```python
from build123d import *

# Parameters (mm, degrees)
F0_W     = 203.2
F0_H     = 15.875
F1_DEPTH = 342.9
F3_DEPTH = 342.9
F4_W     = 15.875
F4_H     = 5.55625
F5_DEPTH = 203.2


with BuildPart() as f1:
    # F0 (on Front) → F1 (new body)
    with BuildSketch(Plane.XZ):
        with Locations((101.6, 7.9375)):
            Rectangle(F0_W, F0_H)
    extrude(amount=F1_DEPTH)

    # F2 (on face) → F3 (cut, through all)
    with BuildSketch(Plane.XZ.offset(342.9)):
        Polygon((32.54375, 5.55625), (32.54375, 0), (56.35625, 0), (56.35625, 5.55625), (53.975, 5.55625), (53.975, 3.96875), (34.925, 3.96875), (34.925, 5.55625), align=None)
        Polygon((170.65625, 5.55625), (168.275, 5.55625), (168.275, 3.96875), (149.225, 3.96875), (149.225, 5.55625), (146.84375, 5.55625), (146.84375, 0), (170.65625, 0), align=None)
    extrude(amount=-F3_DEPTH, mode=Mode.SUBTRACT)

    # F4 (on face) → F5 (cut, through all)
    with BuildSketch(Plane(origin=(0, 0, 0), x_dir=(0, -1, 0), z_dir=(-1, 0, 0))):
        with Locations((20.6375, 13.096875)):
            Rectangle(F4_W, F4_H)
        with Locations((322.2625, 13.096875)):
            Rectangle(F4_W, F4_H)
    extrude(amount=-F5_DEPTH, mode=Mode.SUBTRACT)


solid = f1.part
```
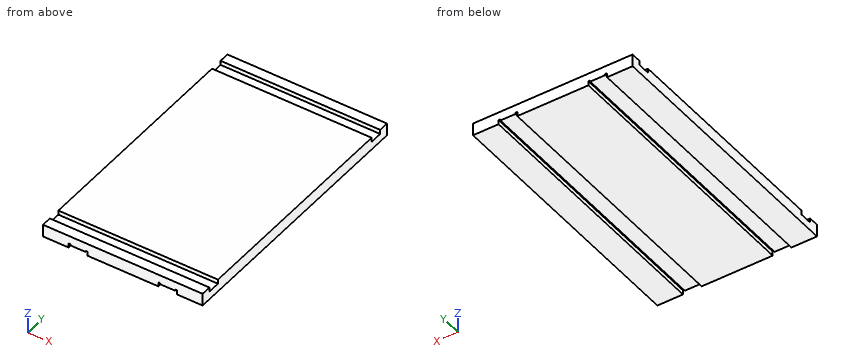
For this review, take the finished solid that the model builds, in its own axes (mm). Coordinates: 2 decimals unless noted, no trailing zeros. Write each loop counter-clockwise with the first axis right and the second up, starting at its lowest first coordinate (ties: lowest second). Pieces come first, ordered by that corner, then holes. Notation, with made-up numbers: (65, 1.5) -> (86, 1.5) arc R23 ccw to (86, 22.5) -> close; hole circle Ø9 at (47.5, -27). An arc over 180 degrees is marked (long way). Put each result on its own line as item: value.
Q1. Clearance check with flat-ended pins moving along their axes: pin 1 Ø8 at (x, y) = (114, -321) entering from +Z; pin 2 Ø1.9 at (x, y) = (54.5, -171) entering from -Z; pin 3 Ø1.9 at (x, y) = (169.5, -219) entering from -Z. State where each tip first meets the part, or that it passes through.
From the geometry:
pin 1: stops at z = 10.32
pin 2: stops at z = 3.97
pin 3: stops at z = 5.56
Q2. Wall thickness on L1, parallel to X at y = -265, z = 3; L2, parallel to X at y = -210, z = 4.25 (3 decimals); L3, parallel to Y at x = 50, z = 12.5 (3 decimals): over which ranges is each line inside the solid? List them lowest first.
From the geometry:
L1: x = 0 to 32.54, 56.36 to 146.84, 170.66 to 203.2
L2: x = 0 to 32.544, 34.925 to 53.975, 56.356 to 146.844, 149.225 to 168.275, 170.656 to 203.2
L3: y = -342.9 to -330.2, -314.325 to -28.575, -12.7 to 0
Q3. Take a section at B-B, the plane x = 154. State the section outline as (y, z) points (3 decimals).
From the geometry:
outline: (-342.9, 3.969) -> (0, 3.969) -> (0, 15.875) -> (-12.7, 15.875) -> (-12.7, 10.319) -> (-28.575, 10.319) -> (-28.575, 15.875) -> (-314.325, 15.875) -> (-314.325, 10.319) -> (-330.2, 10.319) -> (-330.2, 15.875) -> (-342.9, 15.875) -> close
Q4. Take a section at C-C, the plane x = 190. State the section outline as (y, z) points (3 decimals).
From the geometry:
outline: (-342.9, 0) -> (0, 0) -> (0, 15.875) -> (-12.7, 15.875) -> (-12.7, 10.319) -> (-28.575, 10.319) -> (-28.575, 15.875) -> (-314.325, 15.875) -> (-314.325, 10.319) -> (-330.2, 10.319) -> (-330.2, 15.875) -> (-342.9, 15.875) -> close
Q5. Take a section at D-D, the plane y = -22. State the section outline as (x, z) points (3 decimals).
From the geometry:
outline: (0, 0) -> (32.544, 0) -> (32.544, 5.556) -> (34.925, 5.556) -> (34.925, 3.969) -> (53.975, 3.969) -> (53.975, 5.556) -> (56.356, 5.556) -> (56.356, 0) -> (146.844, 0) -> (146.844, 5.556) -> (149.225, 5.556) -> (149.225, 3.969) -> (168.275, 3.969) -> (168.275, 5.556) -> (170.656, 5.556) -> (170.656, 0) -> (203.2, 0) -> (203.2, 10.319) -> (0, 10.319) -> close
Q6. Take a section at A-A, the plane y = -291. State the section outline as (x, z) points (3 decimals).
From the geometry:
outline: (0, 0) -> (32.544, 0) -> (32.544, 5.556) -> (34.925, 5.556) -> (34.925, 3.969) -> (53.975, 3.969) -> (53.975, 5.556) -> (56.356, 5.556) -> (56.356, 0) -> (146.844, 0) -> (146.844, 5.556) -> (149.225, 5.556) -> (149.225, 3.969) -> (168.275, 3.969) -> (168.275, 5.556) -> (170.656, 5.556) -> (170.656, 0) -> (203.2, 0) -> (203.2, 15.875) -> (0, 15.875) -> close
